Build history of the part. All positions in model axes, mm. A direction names the side the tool comes from. Give positions to 0.01 mm unless a question says otherwise; leave off trailing zeros. Loops run counter-clockwise (first coordinate to the right, second up) from the corner with the lowest first, then second, coordinate; pieces in that order, holes last.
1) Wall check: line 1 (X direction, y = 0.9, z = -32); line 2 (X direction, y = -0.1, z = -40). Give the ranges that are in metal, low to high.
2) Two-plate mould, pull along Z, no slides. Class faces 3 (the cylindrical face through (0.401, 1.806, 60.246)), 4 (the flat face through (0, 0, 62.3)), 5 (the cylindrical face through (0, -2, 1)): +Z half, -Z half, draft (parallel to the pull), parting line (faces both ways), or undercut.
3) Band-saw the part on A-A on z = -12. List the corners of the cut face in (x, y).
4) Flat gauge pins, fed straight in: P1, Ø1, axis at x = -1, z = -26, coming from the -Y side; P2, Ø1.5, axis at y = -1.5, z = -46, coming from the -X side; P3, Ø1, axis at x = -1.5, z = 11.5, coming from the -Y side. Where does each tip first touch, or does it go through?
5) 3-axis set-ups, long thin cutter, end or side, ignore diameter. For faces 1 (the cylindrical face through (0.401, 1.806, -60.254)), 2 (the cylindrical face through (0, -2, 61)): which of +Z, -Z, +X, -X, +Y, -Y reach the whole face in a straight line?
```python
from build123d import *

# Parameters (mm, degrees)
SKIZZE1_R                       = 2
AUFSATZ_LINEAR_AUSTRAGEN1_DEPTH = 62.3
SKIZZE7_W                       = 0.5
SKIZZE7_H                       = 0.15
FASE1_SIZE                      = 0.2


with BuildPart() as part:
    # Skizze1 → Aufsatz-Linear austragen1 (new, symmetric)
    with BuildSketch(Plane.XY):
        Circle(SKIZZE1_R)
    extrude(amount=AUFSATZ_LINEAR_AUSTRAGEN1_DEPTH, both=True)

    # Skizze7 → Schnitt-Rotation1 (revolve, cut)
    with BuildSketch(Plane(origin=(0, 0, 0), x_dir=(0, 0, -1), z_dir=(1, 0, 0)), mode=Mode.PRIVATE) as schnitt_rotation1_sk:
        with Locations((-60.25, 1.925)):
            Rectangle(SKIZZE7_W, SKIZZE7_H)
        with Locations((60.25, 1.925)):
            Rectangle(SKIZZE7_W, SKIZZE7_H)
    revolve(schnitt_rotation1_sk.sketch.rotate(Axis((0, 0, -62.3), (0, 0, 1)), 90), axis=Axis((0, 0, -62.3), (0, 0, 1)), mode=Mode.SUBTRACT)

    # Fase1
    fase1_edges = [part.edges().sort_by_distance(p)[0] for p in [
        (-2, 0, -62.3),
        (-2, 0, 62.3),
    ]]
    chamfer(fase1_edges, length=FASE1_SIZE)


solid = part.part
```
Findings below:
1. line 1: x = -1.79 to 1.79
1. line 2: x = -2 to 2
2. face 3: undercut
2. face 4: +Z half
2. face 5: draft
3. outline: circle Ø4 at (0, 0)
4. P1: stops at y = -1.94
4. P2: stops at x = -1.85
4. P3: stops at y = -1.73
5. face 1: none
5. face 2: +Z, -Z
